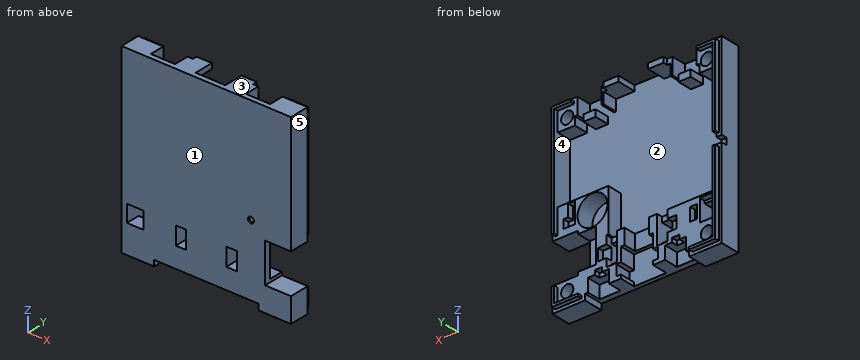
```python
from build123d import *

# Parameters (mm, degrees)
SKETCH_1_W           = 56.974706629
SKETCH_1_H           = 61.774716789
EXTRUDE_1_DEPTH      = 6.7
SKETCH_2_W           = 8.669316727
SKETCH_2_H           = 13.354025908
CUT_EXTRUDE_1_DEPTH  = 57.923066884
SKETCH_3_W           = 6.025008901
SKETCH_3_H           = 11.3000508
CUT_EXTRUDE_2_DEPTH  = 4.7
SKETCH_4_R           = 5.03
CUT_EXTRUDE_3_DEPTH  = 6
SKETCH_5_R           = 1
CUT_EXTRUDE_4_DEPTH  = 57.923066884
CUT_EXTRUDE_5_DEPTH  = 2
CUT_EXTRUDE_6_DEPTH  = 2
SKETCH_8_W           = 3.513995428
SKETCH_8_H           = 6.075560276
CUT_EXTRUDE_7_DEPTH  = 57.923066884
SKETCH_9_W           = 7.063042926
SKETCH_9_H           = 4.362369824
CUT_EXTRUDE_8_DEPTH  = 4.7
SKETCH_10_W          = 2.4499365
SKETCH_10_H          = 1.42002794
CUT_EXTRUDE_9_DEPTH  = 2
SKETCH_11_W          = 35.063093726
SKETCH_11_H          = 2
CUT_EXTRUDE_10_DEPTH = 57.923066884
CUT_EXTRUDE_11_DEPTH = 5.3
SKETCH_13_W          = 8.286080772
SKETCH_13_H          = 5.236537973
CUT_EXTRUDE_12_DEPTH = 4.2
SKETCH_14_W          = 2.359613919
SKETCH_14_H          = 4.479603759
SKETCH_14_W_2        = 5.594310389
SKETCH_14_H_2        = 7.413106427
CUT_EXTRUDE_13_DEPTH = 2
SKETCH_15_W          = 5.594310389
SKETCH_15_H          = 5.734010668
CUT_EXTRUDE_14_DEPTH = 57.923066884
CUT_EXTRUDE_15_DEPTH = 5
SKETCH_18_W          = 8.154025908
SKETCH_18_H          = 6.040749301
CUT_EXTRUDE_16_DEPTH = 5
SKETCH_19_W          = 2.683012447
SKETCH_19_H          = 2.737564136
SKETCH_19_W_2        = 2.913081027
SKETCH_19_W_3        = 2.717012954
SKETCH_19_H_2        = 2.737561596
SKETCH_19_W_4        = 2.913081026
CUT_EXTRUDE_17_DEPTH = 5
EXTRUDE_4_DEPTH      = 1.5
SKETCH_25_R          = 2.05
CUT_EXTRUDE_18_DEPTH = 5
CUT_EXTRUDE_19_REACH = 74.547
SKETCH_26_W          = 2.2
SKETCH_26_H          = 2


with BuildPart() as part:
    # 草图1 → 凸台-拉伸1 (new body)
    with BuildSketch(Plane(origin=(0, 0, 0), x_dir=(1, 0, 0), z_dir=(0, 1, 0))):
        with Locations((6.805733636, 13.268542196)):
            Rectangle(SKETCH_1_W, SKETCH_1_H)
    extrude(amount=EXTRUDE_1_DEPTH)

    # 草图2 → 切除-拉伸1 (cut, through all)
    with BuildSketch(Plane(origin=(0, 6.7, 0), x_dir=(1, 0, 0), z_dir=(0, 1, 0))):
        with Locations((30.958428588, 29.168521876)):
            Rectangle(SKETCH_2_W, SKETCH_2_H)
    extrude(amount=-CUT_EXTRUDE_1_DEPTH, mode=Mode.SUBTRACT)

    # 草图3 → 切除-拉伸2 (cut)
    with BuildSketch(Plane(origin=(0, 6.7, 0), x_dir=(1, 0, 0), z_dir=(0, 1, 0))):
        with Locations((23.611265774, 29.168534576)):
            Rectangle(SKETCH_3_W, SKETCH_3_H)
    extrude(amount=-CUT_EXTRUDE_2_DEPTH, mode=Mode.SUBTRACT)

    # 草图4 → 切除-拉伸3 (cut)
    with BuildSketch(Plane(origin=(0, 6.7, 0), x_dir=(1, 0, 0), z_dir=(0, 1, 0))):
        with Locations(Location((21.805764117, 18.168422815, 0), (0, 0, 270))):
            Circle(SKETCH_4_R)
    extrude(amount=-CUT_EXTRUDE_3_DEPTH, mode=Mode.SUBTRACT)

    # 草图5 → 切除-拉伸4 (cut, through all)
    with BuildSketch(Plane(origin=(0, 6.7, 0), x_dir=(1, 0, 0), z_dir=(0, 1, 0))):
        with Locations(Location((21.805764117, 18.168422815, 0), (0, 0, 270))):
            Circle(SKETCH_5_R)
    extrude(amount=-CUT_EXTRUDE_4_DEPTH, mode=Mode.SUBTRACT)

    # 草图6 → 切除-拉伸5 (cut)
    with BuildSketch(Plane(origin=(0, 6.7, 0), x_dir=(1, 0, 0), z_dir=(0, 1, 0))):
        Polygon((29.999071203, 13.131206661), (27.61248243, 13.131206661), (27.61248243, 20.17096536), (31.608192362, 20.17096536), (31.608192362, 17.212011843), (29.999071203, 17.212011843), align=None)
    extrude(amount=-CUT_EXTRUDE_5_DEPTH, mode=Mode.SUBTRACT)

    # 草图7 → 切除-拉伸6 (cut)
    with BuildSketch(Plane(origin=(0, 6.7, 0), x_dir=(1, 0, 0), z_dir=(0, 1, 0))):
        Polygon((13.535748877, 27.373568866), (17.049744305, 27.373568866), (17.049744305, 30.131239681), (19.999050883, 30.131239681), (19.999050883, 34.20591583), (17.049744305, 34.20591583), (17.049744305, 36.963586646), (13.535748877, 36.963586646), align=None)
        Polygon((0.049708745, 27.373568866), (0.049708745, 36.963586646), (-3.464286683, 36.963586646), (-3.464286683, 34.20591583), (-6.38758361, 34.20591583), (-6.38758361, 30.131239681), (-3.464286683, 30.131239681), (-3.464286683, 27.373568866), align=None)
    extrude(amount=-CUT_EXTRUDE_6_DEPTH, mode=Mode.SUBTRACT)

    # 草图8 → 切除-拉伸7 (cut, through all)
    with BuildSketch(Plane(origin=(0, 6.7, 0), x_dir=(1, 0, 0), z_dir=(0, 1, 0))):
        with Locations((15.292746591, 32.16678949)):
            Rectangle(SKETCH_8_W, SKETCH_8_H)
        with Locations((-1.707288969, 32.16678949)):
            Rectangle(SKETCH_8_W, SKETCH_8_H)
    extrude(amount=-CUT_EXTRUDE_7_DEPTH, mode=Mode.SUBTRACT)

    # 草图9 → 切除-拉伸8 (cut)
    with BuildSketch(Plane(origin=(0, 6.7, 0), x_dir=(1, 0, 0), z_dir=(0, 1, 0))):
        with Locations((19.805886037, 39.974715678)):
            Rectangle(SKETCH_9_W, SKETCH_9_H)
        with Locations((-6.194164763, 39.974715678)):
            Rectangle(SKETCH_9_W, SKETCH_9_H)
    extrude(amount=-CUT_EXTRUDE_8_DEPTH, mode=Mode.SUBTRACT)

    # 草图10 → 切除-拉伸9 (cut)
    with BuildSketch(Plane(origin=(0, 6.7, 0), x_dir=(1, 0, 0), z_dir=(0, 1, 0))):
        with Locations((19.805759037, 37.083516796)):
            Rectangle(SKETCH_10_W, SKETCH_10_H)
        with Locations((-6.194291763, 37.083516796)):
            Rectangle(SKETCH_10_W, SKETCH_10_H)
    extrude(amount=-CUT_EXTRUDE_9_DEPTH, mode=Mode.SUBTRACT)

    # 草图11 → 切除-拉伸10 (cut, through all)
    with BuildSketch(Plane(origin=(0, 6.7, 0), x_dir=(1, 0, 0), z_dir=(0, 1, 0))):
        with Locations((6.805860637, 43.15590059)):
            Rectangle(SKETCH_11_W, SKETCH_11_H)
    extrude(amount=-CUT_EXTRUDE_10_DEPTH, mode=Mode.SUBTRACT)

    # 草图12 → 切除-拉伸11 (cut)
    with BuildSketch(Plane(origin=(0, 6.7, 0), x_dir=(1, 0, 0), z_dir=(0, 1, 0))):
        Polygon((12.21261705, 42.15590059), (12.21261705, 40.952697644), (13.78261959, 40.952697644), (13.78261959, 37.307917354), (12.21261705, 37.307917354), (12.21261705, 32.60558055), (1.398596223, 32.60558055), (1.398596223, 37.333317405), (-0.171406318, 37.333317405), (-0.171406318, 40.882923704), (1.400885865, 40.882923704), (1.400885865, 42.15590059), align=None)
    extrude(amount=-CUT_EXTRUDE_11_DEPTH, mode=Mode.SUBTRACT)

    # 草图13 → 切除-拉伸12 (cut)
    with BuildSketch(Plane(origin=(0, 6.7, 0), x_dir=(1, 0, 0), z_dir=(0, 1, 0))):
        with Locations((6.869233764, 29.987311564)):
            Rectangle(SKETCH_13_W, SKETCH_13_H)
    extrude(amount=-CUT_EXTRUDE_12_DEPTH, mode=Mode.SUBTRACT)

    # 草图14 → 切除-拉伸13 (cut)
    with BuildSketch(Plane(origin=(0, 6.7, 0), x_dir=(1, 0, 0), z_dir=(0, 1, 0))):
        with Locations((-12.194304463, 31.668577756)):
            Rectangle(SKETCH_14_W, SKETCH_14_H)
        with Locations((-17.084464483, 31.668577756)):
            Rectangle(SKETCH_14_W_2, SKETCH_14_H_2)
    extrude(amount=-CUT_EXTRUDE_13_DEPTH, mode=Mode.SUBTRACT)

    # 草图15 → 切除-拉伸14 (cut, through all)
    with BuildSketch(Plane(origin=(0, 6.7, 0), x_dir=(1, 0, 0), z_dir=(0, 1, 0))):
        with Locations((-17.084464483, 31.668653956)):
            Rectangle(SKETCH_15_W, SKETCH_15_H)
    extrude(amount=-CUT_EXTRUDE_14_DEPTH, mode=Mode.SUBTRACT)

    # 草图16 → 切除-拉伸15 (cut)
    with BuildSketch(Plane(origin=(0, 6.7, 0), x_dir=(1, 0, 0), z_dir=(0, 1, 0))):
        Polygon((16.449751925, 27.39556785), (-19.881619678, 27.39556785), (-19.881619678, -9.340502762), (-4.46782745, -9.340502762), (-4.46782745, -15.818816199), (1.788733383, -15.818816199), (1.788733383, -17.618816199), (11.788733383, -17.618816199), (11.788733383, -15.818816199), (18.045294216, -15.818816199), (18.045294216, -9.340505302), (33.493086951, -9.340505302), (33.493086951, 12.913538386), (16.449751925, 12.913538386), align=None)
    extrude(amount=-CUT_EXTRUDE_15_DEPTH, mode=Mode.SUBTRACT)

    # 草图18 → 切除-拉伸16 (cut)
    with BuildSketch(Plane(origin=(0, 6.7, 0), x_dir=(1, 0, 0), z_dir=(0, 1, 0))):
        with Locations((-9.194172383, -14.598441549)):
            Rectangle(SKETCH_18_W, SKETCH_18_H)
        with Locations((22.805893657, -14.598441549)):
            Rectangle(SKETCH_18_W, SKETCH_18_H)
    extrude(amount=-CUT_EXTRUDE_16_DEPTH, mode=Mode.SUBTRACT)

    # 草图19 → 切除-拉伸17 (cut)
    with BuildSketch(Plane(origin=(0, 6.7, 0), x_dir=(1, 0, 0), z_dir=(0, 1, 0))):
        with Locations((-5.809333674, -10.70928483)):
            Rectangle(SKETCH_19_W, SKETCH_19_H)
        with Locations((-12.694299384, -10.70928483)):
            Rectangle(SKETCH_19_W_2, SKETCH_19_H)
        with Locations((19.403800693, -10.7092861)):
            Rectangle(SKETCH_19_W_3, SKETCH_19_H_2)
        with Locations((26.305766657, -10.7092861)):
            Rectangle(SKETCH_19_W_4, SKETCH_19_H_2)
    extrude(amount=-CUT_EXTRUDE_17_DEPTH, mode=Mode.SUBTRACT)

    # 草图24 → 凸台-拉伸4 (add)
    with BuildSketch(Plane(origin=(0, 6.7, 0), x_dir=(1, 0, 0), z_dir=(0, 1, 0))):
        Polygon((-11.825686226, 42.35590059), (-19.881619678, 42.35590059), (-19.881619678, 15.076541942), (-20.681619678, 15.076541942), (-20.681619678, 43.15590059), (-11.825686226, 43.15590059), align=None)
        Polygon((-19.881619678, -15.818816199), (-14.371185337, -15.818816199), (-14.371185337, -16.618816199), (-20.681619678, -16.618816199), (-20.681619678, 10.876541942), (-19.881619678, 10.876541942), align=None)
        Polygon((33.493086951, -15.818816199), (33.493086951, 21.391508922), (34.293086951, 21.391508922), (34.293086951, -16.618816199), (27.982906611, -16.618816199), (27.982906611, -15.818816199), align=None)
        Polygon((33.493086951, 36.94553483), (33.493086951, 42.35590059), (25.4374075, 42.35590059), (25.4374075, 43.15590059), (34.293086951, 43.15590059), (34.293086951, 36.94553483), align=None)
        Polygon((1.788733383, -16.618816199), (1.788733383, -15.818816199), (-3.313915843, -15.818816199), (-3.313915843, -17.618816199), (1.788733383, -17.618816199), align=None)
        Polygon((11.788733383, -16.618816199), (11.788733383, -15.818816199), (16.925383116, -15.818816199), (16.925383116, -17.618816199), (11.788733383, -17.618816199), align=None)
    extrude(amount=EXTRUDE_4_DEPTH)

    # 草图25 → 切除-拉伸18 (cut)
    with BuildSketch(Plane(origin=(0, 6.7, 0), x_dir=(1, 0, 0), z_dir=(0, 1, 0))):
        with Locations(Location((30.305781897, -12.631511144, 0), (0, 0, 270))):
            Circle(SKETCH_25_R)
        with Locations(Location((-16.694314623, 39.168592996, 0), (0, 0, 270))):
            Circle(SKETCH_25_R)
        with Locations(Location((-16.694314623, -12.631511144, 0), (0, 0, 270))):
            Circle(SKETCH_25_R)
        with Locations(Location((30.305781897, 39.168592996, 0), (0, 0, 270))):
            Circle(SKETCH_25_R)
    extrude(amount=-CUT_EXTRUDE_18_DEPTH, mode=Mode.SUBTRACT)

    # 草图26 → 切除-拉伸19 (cut, up to next)
    with BuildSketch(Plane.ZY.offset(21.681619678), mode=Mode.PRIVATE) as cut_extrude_19_sk1:
        with Locations((-12.976541942, 5.7)):
            Rectangle(SKETCH_26_W, SKETCH_26_H)
    cut_extrude_19_tool1 = extrude(cut_extrude_19_sk1.sketch, amount=-CUT_EXTRUDE_19_REACH, mode=Mode.PRIVATE) & part.part
    add(cut_extrude_19_tool1.solids().sort_by_distance((-21.68162, 5.7, -12.976542))[0], mode=Mode.SUBTRACT)


solid = part.part
```
Verification items for the finished model (mm, model axes). Face numbers are marked on the shaded views. A direction names the side the tool comes from. Round coordinates to 2 decimals unless told otherwise and drop trailing zeros. Write each loop counter-clockwise with the first axis right and the second up, starting at its lowest first coordinate (ties: lowest second). Pieces come first, ordered by that corner, then holes. Notation, with made-up numbers: (75.5, -18.5) - (128.5, -18.5) arc R15 cw to (128.5, 10.5) - close; hole circle Ø10 at (-15.75, -12.75). An arc over 180 degrees is marked (long way). Answer as a JSON object with one key per item and string values. Group by question number.
Q1. Section check A-A, the plane y = 7.5. Give the number of separate pieces and of enclosed holes in the cut face, plus the area to 3 significant figures.
Q2. Section check D-D, the plane z = 4. Enter the section's corners in (x, y), plus the area to 3 significant figures.
Q3. Mould release check, pull along Z, two halves, no side actions. Record for the marked faces 1, 2 and 3: released by +Z, released by -Z, zero draft, split by the parting line, or undercut.
Q4. Tool access check on the marked faces 4 and 5. Record the directions out of +Z, -Z, +X, -X, +Y, -Y that give a thin tool (end or side, any length) a straight path to the whole face; none if there is none.
Q5. Go/stop test with flat-tipped pins: pin 1 Ø2 at (x, y) = (4, 2) entering from -Z; pin 2 Ø1.2 at (y, z) = (7.5, 17) entering from +X; pin 3 Ø0.5 at (x, z) = (-4.5, 15.5) entering from +Y. Record where each tip stops, or that it passes through.
Q6. Thickness scan on line 1 (X direction, y = 6.5, z = -30); line 2 (Z direction, x = -1, y = 4.5); line 3 (X direction, y = 5.25, z = -35). Record the ranges inside material, lowest first.
Found:
{
 "1": {"separate pieces": "6", "enclosed holes": "0", "area": "120 mm^2"},
 "2": {"outline": "(-21.68, 0) - (35.29, 0) - (35.29, 6.7) - (34.29, 6.7) - (34.29, 8.2) - (33.49, 8.2) - (33.49, 1.7) - (-19.88, 1.7) - (-19.88, 8.2) - (-20.68, 8.2) - (-20.68, 6.7) - (-21.68, 6.7) - close", "area": "117 mm^2"},
 "3": {"face 1": "zero draft", "face 2": "undercut", "face 3": "released by +Z"},
 "4": {"face 4": "+Y", "face 5": "+Z, -Z, +X, +Y, -Y"},
 "5": {"pin 1": "stops at z = -42.16", "pin 2": "stops at x = 34.29", "pin 3": "stops at y = 6.7"},
 "6": {"line 1": "x = -21.68 to -19.88, -14.29 to -13.37, -11.01 to -3.46, 0.05 to 2.73, 11.01 to 13.54, 17.05 to 20.6", "line 2": "z = -42.16 to -35.2, -29.13 to -27.4, 15.82 to 17.62", "line 3": "x = -21.68 to -19.88, -14.29 to -3.46, 0.05 to 1.4, 12.21 to 13.54, 17.05 to 26.62"}
}
